Drawing for the job (mm, zero at the part's lowest x, y, z). Coordinates: 2 decimals unless noted, no trailing zeros. Loops run counter-clockwise (first coordinate to the right, second up) from the corner with the lowest first, then second, coordinate; pieces in that order, holes last.
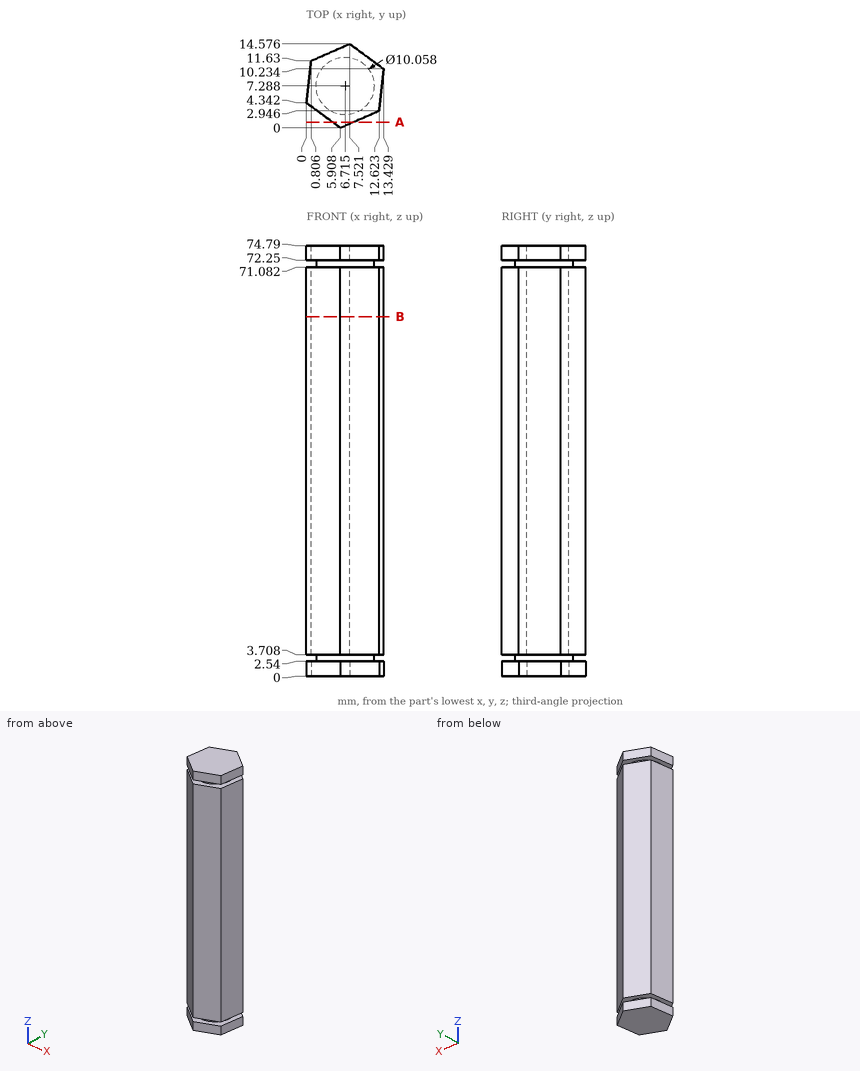
Q1. Drop flat-ended pins along their axis: P1, Ø6, axis at x = 11.5, z = 58.5, coming from the +Y side (1 decimal); P2, Ø3, axis at y = 12, z = 21, coming from the -X side; P3, Ø4, axis at y = 8, z = 43, coming from the +X side. Give the stop position or say it passes through.
Q2. Saw through at B-B (z = 62.5). List the corners of the cut face in (x, y) (1 decimal), plus the area to 3 significant figures.
Q3. Probe line 1 (Z direction, x = 7.5, y = 12.75); line 2 (Y direction, x = 10, z = 17.5) (1 decimal); line 3 (Y direction, x = 8.75, z = 65.5) (1 decimal). List the from-to ranges inside material, lowest first.
Q4. Saw through at A-A (y = 1). List the corners of the cut face in (x, z).
Checked values:
1. P1: stops at y = 13.9
1. P2: stops at x = 0.68
1. P3: stops at x = 13.4
2. outline: (0, 4.3) - (5.9, 0) - (12.6, 2.9) - (13.4, 10.2) - (7.5, 14.6) - (0.8, 11.6) - close
2. area: 140 mm2
3. line 1: z = 0 to 2.54, 3.71 to 71.08, 72.25 to 74.79
3. line 2: y = 1.8 to 12.8
3. line 3: y = 1.2 to 13.7
4. outline: (4.55, 0) - (8.19, 0) - (8.19, 2.54) - (4.55, 2.54) - close; (4.55, 3.71) - (8.19, 3.71) - (8.19, 71.08) - (4.55, 71.08) - close; (4.55, 72.25) - (8.19, 72.25) - (8.19, 74.79) - (4.55, 74.79) - close
